Check sheet for the modelled part. Datum: model origin and axes. Units: mm. A direction names the side the tool comes from. Coordinates: 2 decimals unless noted, no trailing zeros. Loops run counter-clockwise (first coordinate to the right, second up) from the corner with the lowest first, then second, coordinate; pieces in that order, holes last. Notation, with made-up numbers: (-14.75, -30) -> (0.25, -30) arc R14 cw to (0.25, -24) -> close; hole circle Ø9 at (-29.5, -11). An arc over 180 degrees is marked (long way). Use CSV: the item, a comma, the result in double quotes.
Autodesk Inventor part; units mm, degrees
ref_plane "YZ Plane" through (0, 0, 0) normal (1, 0, 0) x (0, 1, 0)
ref_plane "XZ Plane" through (0, 0, 0) normal (0, 1, 0) x (-1, 0, 0)
ref_plane "XY Plane" through (0, 0, 0) normal (0, 0, 1) x (1, 0, 0)
sketch "スケッチ1" plane through (0, 0, 0) normal (0, 1, 0) x (-1, 0, 0)
  line L0 (-10, -9.5) -> (10, -9.5)
  line L1 (10, -9.5) -> (10, 9.5)
  line L2 (10, 9.5) -> (-10, 9.5)
  line L3 (-10, 9.5) -> (-10, -9.5)
  line L4 (-10, -9.5) -> (10, 9.5) construction
  line L5 (10, -9.5) -> (-10, 9.5) construction
  point P0 (0, 0)
  dimension "d0" = 20
  dimension "d1" = 19
extrude "プレート1" add sketch "スケッチ1" along normal blind 3
sketch "スケッチ5" plane through (0, 3, 0) normal (0, 1, 0) x (1, 0, 0)
  point P0 (0, 0)
sketch "スケッチ6" plane through (-10.7765, 3.1022, 9.5) normal (-0.258819, -0.9659258, 0) x (0.9659258, -0.258819, 0)
  line L0 (0, -19) -> (0, 0)
  line L1 (0, 0) -> (-18.2101, 0)
  line L2 (-18.2101, 0) -> (-18.2101, -19)
  line L3 (-18.2101, -19) -> (0, -19)
edge flange "フランジ3" height 19 angle 15 thickness 3 bend radius 3 thickness toward (-0.258819, -0.9659258, 0) relief tear relief width 3 relief depth 1.5 edges at (-10, 3, 0) wall of the first edge with corners at (-10.7765, 3.1022, -9.5) (-10.7765, 3.1022, 9.5) (-28.366, 7.8153, 9.5) (-28.366, 7.8153, -9.5)
bend "曲げ3"
corner "コーナー3"
sketch "スケッチ7" plane through (-29.919, 5.0198, 9.5) normal (0, 1, 0) x (1, 0, 0)
  line L0 (0, -19) -> (0, 0)
  line L1 (0, 0) -> (-3.0801, 0)
  line L2 (-3.0801, 0) -> (-3.0801, -19)
  line L3 (-3.0801, -19) -> (0, -19)
edge flange "フランジ4" height 3.87 angle -15 thickness 3 bend radius 3 thickness toward (0, 1, 0) relief tear relief width 3 relief depth 1.5 edges at (-28.366, 7.8153, 0) wall of the first edge with corners at (-29.919, 5.0198, -9.5) (-29.919, 5.0198, 9.5) (-32.999, 5.0198, 9.5) (-32.999, 5.0198, -9.5)
bend "曲げ4"
corner "コーナー4"
sketch "スケッチ8" plane through (13, -3, -9.5) normal (1, 0, 0) x (0, -1, 0)
  line L0 (0, 19) -> (0, 0)
  line L1 (0, 0) -> (9, 0)
  line L2 (9, 0) -> (9, 19)
  line L3 (9, 19) -> (0, 19)
edge flange "フランジ5" height 15 angle -90 thickness 3 bend radius 3 thickness toward (1, 0, 0) relief tear relief width 3 relief depth 1.5 edges at (10, 3, 0) wall of the first edge with corners at (13, -3, 9.5) (13, -3, -9.5) (13, -12, -9.5) (13, -12, 9.5)
bend "曲げ5"
corner "コーナー5"
sketch "スケッチ9" plane through (-35.999, 2.0198, 9.5) normal (-1, 0, 0) x (0, 1, 0)
  line L0 (0, -19) -> (0, 0)
  line L1 (0, 0) -> (-14, 0)
  line L2 (-14, 0) -> (-14, -19)
  line L3 (-14, -19) -> (0, -19)
edge flange "フランジ6" height 20 angle -90 thickness 3 bend radius 3 thickness toward (-1, 0, 0) relief tear relief width 3 relief depth 1.5 edges at (-32.999, 8.0198, 0) wall of the first edge with corners at (-35.999, 2.0198, -9.5) (-35.999, 2.0198, 9.5) (-35.999, -11.9802, 9.5) (-35.999, -11.9802, -9.5)
bend "曲げ6"
corner "コーナー6"
sketch "スケッチ14" plane through (16, -12, 9.5) normal (1, 0, 0) x (0, 0, -1)
  line L0 (4, 6) -> (15, 6)
  arc A0 (15, 2) -> (15, 6) centre (15, 4) ccw
  line L1 (15, 2) -> (4, 2)
  arc A1 (4, 6) -> (4, 2) centre (4, 4) ccw
  line L2 (19, 9) -> (19, 0)
  line L3 (0, 9) -> (0, 0)
  line L4 (0, 0) -> (19, 0)
  point P0 (9.5, 12)
  dimension "d86" = 2
  dimension "d87" = 4
  dimension "d88" = 4
  dimension "d89" = 4
extrude "押し出し6" cut sketch "スケッチ14" against normal blind 100
sketch "スケッチ15" plane through (0, 0, 0) normal (0, -1, 0) x (1, 0, 0)
  line L0 (7.5, -8) -> (-8.5, -8)
  line L1 (-8.5, -8) -> (-8.5, 8)
  line L2 (-8.5, 8) -> (7.5, 8)
  line L3 (7.5, 8) -> (7.5, -8)
  line L4 (7.5, -8) -> (-8.5, 8) construction
  line L5 (-8.5, -8) -> (7.5, 8) construction
  line L6 (-10, -9.5) -> (-10, 9.5)
  point P0 (0, 0)
  point P1 (-0.5, 0)
  point P2 (-0.5, 0)
  dimension "d92" = 16
  dimension "d93" = 16
  dimension "d94" = 9.5
extrude "押し出し7" cut sketch "スケッチ15" against normal blind 1.6
sketch "スケッチ16" plane through (0, 1.6, 0) normal (0, -1, 0) x (1, 0, 0)
  line L0 (-7.5, -7) -> (6.5, -7)
  line L1 (6.5, -7) -> (6.5, 7)
  line L2 (6.5, 7) -> (-7.5, 7)
  line L3 (-7.5, 7) -> (-7.5, -7)
  line L4 (-7.5, -7) -> (6.5, 7) construction
  line L5 (6.5, -7) -> (-7.5, 7) construction
  line L6 (7.5, -8) -> (-8.5, -8)
  line L7 (7.5, 8) -> (7.5, -8)
  point P0 (0, 0)
  point P1 (-0.5, 0)
  point P2 (-0.5, 0)
  point P3 (-0.5, -8)
  point P4 (7.5, 0)
  dimension "d97" = 14
  dimension "d98" = 14
extrude "押し出し8" cut sketch "スケッチ16" against normal blind 1.4
sketch "スケッチ17" plane through (-11.5529, 0.2044, -9.5) normal (-0.258819, -0.9659258, 0) x (0.9659258, -0.258819, 0)
  line L0 (-17.5, 1.5) -> (-1.5, 1.5)
  line L1 (-1.5, 1.5) -> (-1.5, 17.5)
  line L2 (-1.5, 17.5) -> (-17.5, 17.5)
  line L3 (-17.5, 17.5) -> (-17.5, 1.5)
  line L4 (-17.5, 1.5) -> (-1.5, 17.5) construction
  line L5 (-1.5, 1.5) -> (-17.5, 17.5) construction
  line L6 (0, 0) -> (0, 19)
  point P0 (11.2122, 9.5)
  point P1 (-9.5, 9.5)
  point P2 (-9.5, 9.5)
  point P3 (0, 9.5)
  dimension "d101" = 16
  dimension "d102" = 16
  dimension "d103" = 9.5
extrude "押し出し9" cut sketch "スケッチ17" against normal blind 1.6
sketch "スケッチ18" plane through (-11.1388, 1.7499, -9.5) normal (-0.258819, -0.9659258, 0) x (0.9659258, -0.258819, 0)
  line L0 (-16.5, 2.5) -> (-2.5, 2.5)
  line L1 (-2.5, 2.5) -> (-2.5, 16.5)
  line L2 (-2.5, 16.5) -> (-16.5, 16.5)
  line L3 (-16.5, 16.5) -> (-16.5, 2.5)
  line L4 (-16.5, 2.5) -> (-2.5, 16.5) construction
  line L5 (-2.5, 2.5) -> (-16.5, 16.5) construction
  line L6 (-1.5, 17.5) -> (-1.5, 1.5)
  line L7 (-18.2101, 0) -> (0, 0)
  line L8 (-1.5, 1.5) -> (-17.5, 1.5)
  point P0 (11.2122, 9.5)
  point P1 (-9.5, 9.5)
  point P2 (-9.5, 9.5)
  point P3 (-1.5, 9.5)
  point P4 (-9.5, 9.5)
  point P5 (-9.5, 16.5)
  point P6 (-9.105, 0)
  point P7 (-9.5, 1.5)
  dimension "d106" = 14
  dimension "d107" = 14
extrude "押し出し10" cut sketch "スケッチ18" against normal blind 1.4
equation "\"d2\" = Thickness"
equation "\"d29\" = BendReliefWidth"
equation "\"d30\" = BendReliefDepth"
equation "\"d31\" = MinimumRemnant"
equation "\"d32\" = TransitionRadius"
equation "\"d35\" = BendRadius"
equation "\"d36\" = CornerReliefSize"
equation "\"d37\" = GapSize"
equation "\"d38\" = JacobiRadiusSize"
equation "\"d39\" = BendReliefWidth"
equation "\"d40\" = BendReliefDepth"
equation "\"d41\" = MinimumRemnant"
equation "\"d42\" = TransitionRadius"
equation "\"d45\" = BendRadius"
equation "\"d46\" = CornerReliefSize"
equation "\"d47\" = GapSize"
equation "\"d48\" = JacobiRadiusSize"
equation "\"d49\" = BendReliefWidth"
equation "\"d50\" = BendReliefDepth"
equation "\"d51\" = MinimumRemnant"
equation "\"d52\" = TransitionRadius"
equation "\"d55\" = BendRadius"
equation "\"d56\" = CornerReliefSize"
equation "\"d57\" = GapSize"
equation "\"d58\" = JacobiRadiusSize"
equation "\"d59\" = BendReliefWidth"
equation "\"d60\" = BendReliefDepth"
equation "\"d61\" = MinimumRemnant"
equation "\"d62\" = TransitionRadius"
equation "\"d65\" = BendRadius"
equation "\"d66\" = CornerReliefSize"
equation "\"d67\" = GapSize"
equation "\"d68\" = JacobiRadiusSize"
equation "\"BendRadius\" = Thickness"
equation "\"BendReliefWidth\" = Thickness"
equation "\"BendReliefDepth\" = 0.5 * Thickness"
equation "\"CornerReliefSize\" = 4 * Thickness"
equation "\"MinimumRemnant\" = 2 * Thickness"
equation "\"TransitionRadius\" = BendRadius"
equation "\"JacobiRadiusSize\" = BendRadius"
equation "\"GapSize\" = Thickness"
properties part number "thumbkey_plate" material "アルミニウム 6061"
1) Cross-section at A-A on y = -8. Record the boundary of the cut face in (x, z), and give its area (3 significant figures).
Answer below:
outline,"(-39, -9.5) -> (-36, -9.5) -> (-36, -7.5) -> (-39, -7.5) -> close; (-39, 7.5) -> (-36, 7.5) -> (-36, 9.5) -> (-39, 9.5) -> close; (13, -9.5) -> (16, -9.5) -> (16, -7.5) -> (13, -7.5) -> close; (13, 7.5) -> (16, 7.5) -> (16, 9.5) -> (13, 9.5) -> close"
area,"24.0 mm²"
2) Cross-section at D-D on x = -33.5. Record the boundary of the cut face in (y, z), and give its area (3 significant figures).
Answer below:
outline,"(4.98, -9.5) -> (8, -9.5) -> (8, 9.5) -> (4.98, 9.5) -> close"
area,"57.4 mm²"
3) Cross-section at B-B on x = -4.5. Record the boundary of the cut face in (y, z).
Answer below:
outline,"(0, -9.5) -> (3, -9.5) -> (3, -7) -> (1.6, -7) -> (1.6, -8) -> (0, -8) -> close; (0, 8) -> (1.6, 8) -> (1.6, 7) -> (3, 7) -> (3, 9.5) -> (0, 9.5) -> close"
4) Thickness scan on line 1 along X through (y, z) = (1.5, -5.5); line 2 along X through (y, z) = (-5.5, -4); line 3 along X through (y, z) = (2.5, -1.5). Record the ranges inside material, lowest first. Write a range as from..to.
Answer below:
line 1,"x = -39..-36, -12.76..-8.5, 7.5..13.97"
line 2,"x = -39..-36, 13..16"
line 3,"x = -38.98..-35.96, -13.53..-7.5, 6.5..12.4"
5) Access from +Z, -Z, +X, -X, +Y, -Y to the whole of each face (thin tool, end or side, straight path). Record for faces 4 (the flat face through (-8.5, 1, 0)), 5 (the flat face through (7, 3, 0)), 6 (the cylindrical face through (12.14, -0.9, 0.13)), 7 (the flat face through (-37, -10, 0)), 8 (the flat face through (-13.375, 3.065, -0.098)).
Answer below:
face 4,"-Y"
face 5,"+Z, -Z, +X, +Y"
face 6,"+Z, -Z, -Y"
face 7,"+X, -X"
face 8,"+Y"
6) Cross-section at C-C on z = 1.75. Give the number of separate pieces and of enclosed holes in the cut face, and give its area (3 significant figures).
Answer below:
separate pieces,"5"
enclosed holes,"0"
area,"128 mm²"
7) Draft check along Z on faces 1 (the cylindrical face through (-37.5, -8, -7.5)), 2 (the flat face through (-16, 2, -9.5)), 3 (the flat face through (-27.512, 7.587, -0.133)). Enter one of: released by +Z, released by -Z, zero draft, split by the parting line, or undercut.
Answer below:
face 1,"undercut"
face 2,"released by -Z"
face 3,"zero draft"
8) Go/stop test with flat-tipped pins: pin 1 Ø1 at (x, z) = (-20, -7) entering from +Y; pin 2 Ø3.5 at (x, z) = (-38, 1) entering from +Y; pin 3 Ø3.5 at (x, z) = (15, -0.5) entering from +Y. Record where each tip stops, or that it passes through.
Answer below:
pin 1,"stops at y = 5.71"
pin 2,"stops at y = 7.06"
pin 3,"stops at y = 2.04"
